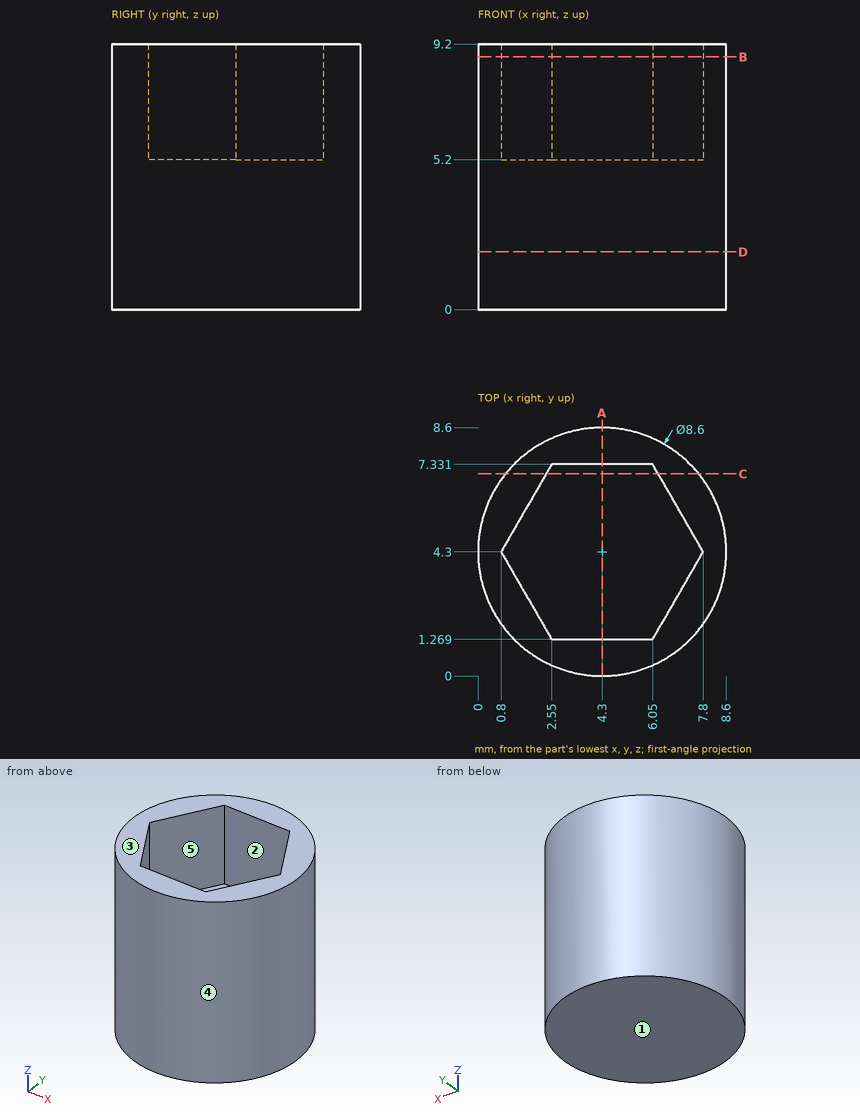
Verification items for this drawing (mm, ordinates from the low corner). A direction names the side the tool comes from. Round coordinates to 2 decimals unless told otherwise and drop trailing zeros. Loops run counter-clockwise (first coordinate to the right, second up) from the corner with the lowest first, then second, coordinate; pieces in that order, holes last. Notation, with made-up numbers: (31, 28.25) - (39, 28.25) arc R9 ccw to (39, 41.25) - close; hole circle Ø7 at (85.25, 12.25). An arc over 180 degrees is marked (long way). Answer as CSV lines item,"result". Start each with the question number.
Item 1: Section check C-C (y = 7). Record the boundary of the cut face in (x, z).
Item 2: Depth check by flat-ended pin: P1, Ø1.5, axis at x = 3, z = 7, coming from the -Y side; P2, Ø3, axis at y = 5, z = 3.5, coming from the -X side; P3, Ø2, axis at y = 7.5, z = 8, coming from the -X side. Enter the tip coordinate at first touch or a pass-through.
Item 3: Set-up check for the marked faces 1 and 2: record each of +Z, -Z, +X, -X, +Y, -Y from which the full face is reachable in a straight line by a thin tool's end or side.
Item 4: Section check B-B (z = 8.75). Record the boundary of the cut face in (x, y).
Item 5: Scan lines: line 1 (Z direction, x = 5, y = 3); line 2 (Y direction, x = 2, z = 7); line 3 (Y direction, x = 4.75, z = 8). Record each from-to range of solid material in increasing order. Write a range as [from, to].
Item 6: Section check A-A (x = 4.3). Record the boundary of the cut face in (y, z), and give its area (3 significant figures).
Item 7: Release check for a two-part mould opening along X. For the marked faces 3, 4 and 5 record: +X half, -X half, draft (parallel to the pull), parting line (faces both ways), or undercut.
Item 8: Section check D-D (z = 2). Record the boundary of the cut face in (x, y).
Report:
1,outline,"(0.95, 0) - (7.65, 0) - (7.65, 9.2) - (6.24, 9.2) - (6.24, 5.2) - (2.36, 5.2) - (2.36, 9.2) - (0.95, 9.2) - close"
2,P1,"stops at y = 0.04"
2,P2,"stops at x = 0"
2,P3,"stops at x = 0.61"
3,face 1,"-Z, +X, -X, +Y, -Y"
3,face 2,"+Z"
4,outline,"circle Ø8.6 at (4.3, 4.3); hole (0.8, 4.3) - (2.55, 1.27) - (6.05, 1.27) - (7.8, 4.3) - (6.05, 7.33) - (2.55, 7.33) - close"
5,line 1,"z = [0, 5.2]"
5,line 2,"y = [0.67, 2.22], [6.38, 7.93]"
5,line 3,"y = [0.02, 1.27], [7.33, 8.58]"
6,outline,"(0, 0) - (8.6, 0) - (8.6, 9.2) - (7.33, 9.2) - (7.33, 5.2) - (1.27, 5.2) - (1.27, 9.2) - (0, 9.2) - close"
6,area,"54.9 mm2"
7,face 3,"draft"
7,face 4,"parting line"
7,face 5,"undercut"
8,outline,"circle Ø8.6 at (4.3, 4.3)"
